from build123d import *

# Parameters (mm, degrees)
BOSS_EXTRUDE1_DEPTH            = 40
SKETCH2_W                      = 40
SKETCH2_H                      = 30
BOSS_EXTRUDE2_DEPTH            = 20
BOSS_EXTRUDE3_DEPTH            = 30
CUT_EXTRUDE1_DEPTH             = 30
SKETCH5_W                      = 70
SKETCH5_H                      = 40
BOSS_EXTRUDE4_DEPTH            = 10
SKETCH6_W                      = 20
SKETCH6_H                      = 20
CUT_EXTRUDE2_DEPTH             = 41
F_10_0_10_DIAMETER_HOLE1_D     = 10
F_10_0_10_DIAMETER_HOLE1_DEPTH = 40
FILLET1_R                      = 20


with BuildPart() as part:
    # Sketch1 → Boss-Extrude1 (new body)
    with BuildSketch(Plane(origin=(0, 0, 0), x_dir=(0, -1, 0), z_dir=(-1, 0, 0))):
        Polygon((-10, -18), (-40, -20), (-10, -20), align=None)
    extrude(amount=-BOSS_EXTRUDE1_DEPTH)

    # Sketch2 → Boss-Extrude2 (add)
    with BuildSketch(Plane(origin=(0, 0, -20), x_dir=(-1, 0, 0), z_dir=(0, 0, -1))):
        with Locations((-20, 25)):
            Rectangle(SKETCH2_W, SKETCH2_H)
    extrude(amount=BOSS_EXTRUDE2_DEPTH)

    # Sketch3 → Boss-Extrude3 (add)
    with BuildSketch(Plane(origin=(40, 0, 0), x_dir=(0, 0, -1), z_dir=(1, 0, 0))):
        Polygon((40, 10), (0, 10), (20, 40), (40, 40), align=None)
    extrude(amount=BOSS_EXTRUDE3_DEPTH)

    # Sketch4 → Cut-Extrude1 (cut)
    with BuildSketch(Plane(origin=(70, 0, 0), x_dir=(0, 0, -1), z_dir=(1, 0, 0))):
        Polygon((20, 40), (0, 10), (30, 10), (30, 30), (40, 30), (40, 40), align=None)
    extrude(amount=-CUT_EXTRUDE1_DEPTH, mode=Mode.SUBTRACT)

    # Sketch5 → Boss-Extrude4 (add)
    with BuildSketch(Plane.XZ.offset(-10)):
        with Locations((35, -20)):
            Rectangle(SKETCH5_W, SKETCH5_H)
    extrude(amount=BOSS_EXTRUDE4_DEPTH)

    # Sketch6 → Cut-Extrude2 (cut, through all)
    with BuildSketch(Plane(origin=(0, 0, -40), x_dir=(-1, 0, 0), z_dir=(0, 0, -1))):
        with Locations((-20, 30)):
            Rectangle(SKETCH6_W, SKETCH6_H)
    extrude(amount=-CUT_EXTRUDE2_DEPTH, mode=Mode.SUBTRACT)

    # Ø10.0 (10) Diameter Hole1
    with Locations(Plane(origin=(0, 0, 0), x_dir=(-1, 0, 0), z_dir=(0, -1, 0))):
        with Locations((-55, 15)):
            Hole(F_10_0_10_DIAMETER_HOLE1_D / 2, depth=F_10_0_10_DIAMETER_HOLE1_DEPTH)

    # Fillet1
    fillet1_edges = [part.edges().sort_by_distance(p)[0] for p in [
        (70, 30, -35),
    ]]
    fillet(fillet1_edges, radius=FILLET1_R)


solid = part.part
The listing builds one solid part. Answer for the finished solid, in the listing's coordinates (mm). A direction names the side the tool comes from. Round coordinates to 2 decimals unless told otherwise and drop trailing zeros. Loops run counter-clockwise (first coordinate to the right, second up) from the corner with the lowest first, then second, coordinate; pieces in that order, holes last. Notation, with made-up numbers: M 88,14 L 94,14 A22 ccw 94,21 Z; hole C 57.25,-28.75 d5. An arc over 180 degrees is marked long. Return JSON: item names as keys, results as strings.
Q1. The mould has two halves that part along Z. Classify faces 1 (the face through (40, 25, -26)), 2 (the face through (51, 5, -12)), 3 (the face through (35, 5, 0)): released by +Z, released by -Z, zero draft, split by the parting line, or undercut.
Results list:
{"face 1": "zero draft", "face 2": "undercut", "face 3": "released by +Z"}
Q2. Each of these flat-tipped pins is pushed along its axis until it touches: pin 1 Ø10 at (y, z) = (33, -13.5) entering from -X; pin 2 Ø24 at (y, z) = (30, -27.5) entering from +X; pin 3 Ø5 at (x, z) = (46, -33) entering from +Y; pin 4 Ø22 at (y, z) = (25, -30.5) entering from +X. Where does it stop, or does it pass through?
Results list:
{"pin 1": "passes through", "pin 2": "stops at x = 68.21", "pin 3": "stops at y = 30", "pin 4": "stops at x = 69.6"}
Q3. Find section D-D, the plane z = -27.5. Determine the outline of the cut face in (x, y).
Results list:
{"outline": "M 0,0 L 70,0 L 70,10 L 40,10 L 40,40 L 30,40 L 30,20 L 10,20 L 10,40 L 0,40 Z"}
Q4. Which of the six approach directions +Z, -Z, +X, -X, +Y, -Y give full straight-line access (tool end or side, diameter ignored) to faces 4 (the face through (10, 30, -29)), 5 (the face through (42, 10, -11)), 6 (the face through (45, 30, -35)), 7 (the face through (19.72, 18.12, -18.54)), 8 (the face through (0, 16, -25))?
Results list:
{"face 4": "+Z, -Z, +Y", "face 5": "+Z, +X, +Y", "face 6": "+Z, -Z, +X, +Y", "face 7": "+Z, +X, -X, +Y", "face 8": "+Z, -Z, -X, +Y, -Y"}
Q5. Find section B-B, the plane x = 55. Determine the outline of the cut face in (y, z), plus the area to 3 significant figures.
Results list:
{"outline": "M 0,-40 L 29.36,-40 L 29.36,-30 L 10,-30 L 10,-20 L 0,-20 Z; M 0,-10 L 10,-10 L 10,0 L 0,0 Z", "area": "494 mm2"}
Q6. Find section A-A, the plane z = -15. Determine the outline of the cut face in (x, y).
Results list:
{"outline": "M 0,0 L 50,0 L 50,10 L 0,10 Z; M 60,0 L 70,0 L 70,10 L 60,10 Z"}
Q7. Find the intervals of material crossed by line 1 along X through (y, z) = (33, -28); line 2 along Z through (x, y) = (55, 3.5); line 3 along Z through (x, y) = (43.5, 19), in increasing order. Write a range as from..to.
Results list:
{"line 1": "x = 0..10, 30..40", "line 2": "z = -40..-20, -10..0", "line 3": "z = -40..-30"}
Q8. Find section C-C, the plane y = 7. Determine the outline of the cut face in (x, z), plus the area to 3 significant figures.
Results list:
{"outline": "M 0,-40 L 70,-40 L 70,0 L 0,0 Z; hole C 55,-15 d10", "area": "2,720 mm2"}
